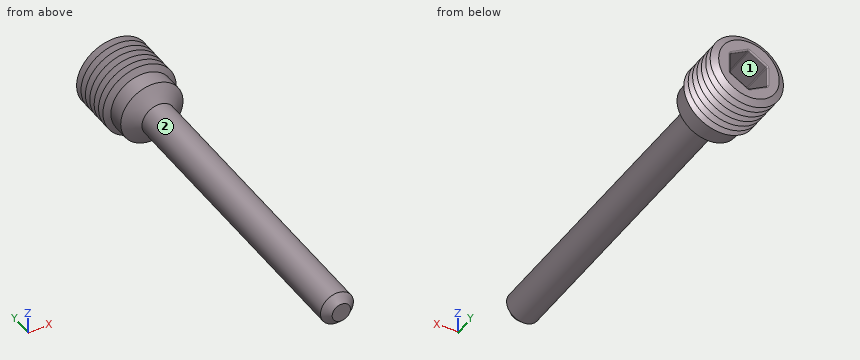
```python
from build123d import *

# Parameters (mm, degrees)
CHAMFER1_SIZE      = 1
CHAMFER2_SIZE      = 0.5
CUT_EXTRUDE1_DEPTH = 7
FILLET1_R          = 0.2


with BuildPart() as part:
    # Sketch1 → Revolve1 (revolve)
    with BuildSketch(Plane.XY):
        Polygon((0, 0), (-2.25, 0), (-2.25, 41.7), (-4.25, 43.2), (-4.25, 45.5), (-5, 45.5), (-5, 52.5), (0, 52.5), align=None)
    revolve(axis=Axis((0, 52.5, 0), (0, -1, 0)))

    # Chamfer1
    chamfer1_edges = [part.edges().sort_by_distance(p)[0] for p in [
        (2.25, 0, 0),
    ]]
    chamfer(chamfer1_edges, length=CHAMFER1_SIZE)

    # Chamfer2
    chamfer2_edges = [part.edges().sort_by_distance(p)[0] for p in [
        (5, 52.5, 0),
    ]]
    chamfer(chamfer2_edges, length=CHAMFER2_SIZE)

    # Sketch2 → Cut-Extrude1 (cut)
    with BuildSketch(Plane(origin=(0, 52.5, 0), x_dir=(1, 0, 0), z_dir=(0, 1, 0))):
        Polygon((0, -2.886751346), (2.5, -1.443375673), (2.5, 1.443375673), (0, 2.886751346), (-2.5, 1.443375673), (-2.5, -1.443375673), align=None)
    extrude(amount=-CUT_EXTRUDE1_DEPTH, mode=Mode.SUBTRACT)

    # Fillet1
    fillet1_edges = [part.edges().sort_by_distance(p)[0] for p in [
        (-1.25, 45.5, 2.165063509),
        (0, 49, 2.886751346),
        (-2.5, 45.5, 0),
        (-2.5, 49, 1.443375673),
        (-1.25, 45.5, -2.165063509),
        (-2.5, 49, -1.443375673),
        (1.25, 45.5, -2.165063509),
        (0, 49, -2.886751346),
        (2.5, 45.5, 0),
        (2.5, 49, -1.443375673),
        (1.25, 45.5, 2.165063509),
        (2.5, 49, 1.443375673),
        (-1.25, 52.5, 2.165063509),
        (1.25, 52.5, 2.165063509),
        (2.5, 52.5, 0),
        (1.25, 52.5, -2.165063509),
        (-1.25, 52.5, -2.165063509),
        (-2.5, 52.5, 0),
    ]]
    fillet(fillet1_edges, radius=FILLET1_R)

    # Sketch3 → Cut-Revolve1 (revolve, cut)
    with BuildSketch(Plane.XY, mode=Mode.PRIVATE) as cut_revolve1_sk:
        Polygon((5, 52), (4.133974596, 51.5), (5, 51), align=None)
        Polygon((5, 51), (4.133974596, 50.5), (5, 50), align=None)
        Polygon((5, 50), (4.133974596, 49.5), (5, 49), align=None)
        Polygon((5, 49), (4.133974596, 48.5), (5, 48), align=None)
        Polygon((5, 48), (4.133974596, 47.5), (5, 47), align=None)
        Polygon((5, 47), (4.133974596, 46.5), (5, 46), align=None)
        Polygon((5, 46), (4.133974596, 45.5), (5, 45), align=None)
        Polygon((5, 53), (4.133974596, 52.5), (5, 52), align=None)
    revolve(cut_revolve1_sk.sketch.rotate(Axis((0, 53.547255409, 0), (0, 1, 0)), 90), axis=Axis((0, 53.547255409, 0), (0, 1, 0)), mode=Mode.SUBTRACT)


solid = part.part
```
Check sheet for the modelled part. Datum: model origin and axes. Units: mm. Face numbers are marked on the shaded views. A direction names the side the tool comes from. Give positions to 0.01 mm unless a question says otherwise; leave off trailing zeros. Order: outer loops, then holes, each group sorted by start corner. A loop starts at its lowest first (then second) coordinate and runs counter-clockwise, first axis right, second up. Notation, with made-up numbers: M 63,6.25 L 74,6.25 A18 ccw 74,39.25 Z; hole C -3.5,88 d6. An arc over 180 degrees is marked long. Answer in a Markdown table with one row per item. Add a question column.
Q1. Access from +Z, -Z, +X, -X, +Y, -Y to the whole of each face (thin tool, end or side, straight path). Record for the marked faces 1 and 2.
Q2. Gauge pin test, flat ends, axial feed: pin 1 Ø1 at (x, y) = (1.5, 9) entering from +Z; pin 2 Ø1.5 at (x, y) = (-2.5, 6.5) entering from -Z; pin 3 Ø1 at (y, z) = (12, -2) entering from +X. Record the tip position at first contact, or that the pin passes through.
Q3. Thickness scan on L1, parallel to Y at x = -0.25, z = 0.75; L2, parallel to Z at x = 0, y = 18.5; L3, parallel to Y at x = -3.75, z = -1.5. Record the ranges inside material, lowest first.
Q4. Sectioned sample at A-A, the plane y = 5.5. Record the boundary of the cut face in (x, z), and give its area (3 significant figures).
Verdict:
| question | item | result |
|---|---|---|
| 1 | face 1 | +Y |
| 1 | face 2 | -Y |
| 2 | pin 1 | z = 2.02 |
| 2 | pin 2 | z = -1.41 |
| 2 | pin 3 | x = 1.68 |
| 3 | L1 | 0 to 45.5 |
| 3 | L2 | -2.25 to 2.25 |
| 3 | L3 | 43.04 to 52.5 |
| 4 | outline | C 0,0 d4.5 |
| 4 | area | 15.9 mm² |
